from build123d import *

# Parameters (mm, degrees)
EXTRUSION1_DEPTH        = 8
ENL_V_MAT_EXTRU_1_DEPTH = 8


with BuildPart() as part:
    # Esquisse1 → Extrusion1 (new body)
    with BuildSketch(Plane.XY):
        with BuildLine():
            Line((1.5, 0), (16.5, 0))
            ThreePointArc((16.5, 0), (17.560660172, 0.439339828), (18, 1.5))
            Line((18, 1.5), (18, 3.5))
            ThreePointArc((18, 3.5), (17.560660172, 4.560660172), (16.5, 5))
            Line((16.5, 5), (1.5, 5))
            ThreePointArc((1.5, 5), (0.439339828, 4.560660172), (0, 3.5))
            Line((0, 3.5), (0, 1.5))
            ThreePointArc((0, 1.5), (0.439339828, 0.439339828), (1.5, 0))
        make_face()
    extrude(amount=EXTRUSION1_DEPTH)

    # Esquisse2 → Enlèv. mat.-Extru.1 (cut)
    with BuildSketch(Plane.XY.offset(8)):
        with BuildLine():
            Line((2.4, 3.095375723), (15.6, 3.095375723))
            ThreePointArc((15.6, 3.095375723), (15.882842712, 2.978218435), (16, 2.695375723))
            Line((16, 2.695375723), (16, 2.495375723))
            ThreePointArc((16, 2.495375723), (15.882842712, 2.21253301), (15.6, 2.095375723))
            Line((15.6, 2.095375723), (2.4, 2.095375723))
            ThreePointArc((2.4, 2.095375723), (2.117157288, 2.21253301), (2, 2.495375723))
            Line((2, 2.495375723), (2, 2.695375723))
            ThreePointArc((2, 2.695375723), (2.117157288, 2.978218435), (2.4, 3.095375723))
        make_face()
    extrude(amount=-ENL_V_MAT_EXTRU_1_DEPTH, mode=Mode.SUBTRACT)


solid = part.part
Read the model definition and answer for the solid it produces. Units are mm, in the model's axes. A direction names the side the tool comes from. Round coordinates to 2 decimals unless told otherwise and drop trailing zeros. Write each loop counter-clockwise with the first axis right and the second up, starting at its lowest first coordinate (ties: lowest second). Pieces come first, ordered by that corner, then holes.
Q1. The mould has two halves that part along Y. Classify faces 1 (the face through (9, 5, 4)), 2 (the face through (9, 0, 4)), 3 (the face through (9, 3.095, 4)): released by +Y, released by -Y, zero draft, split by the parting line, or undercut.
Values:
face 1: released by +Y
face 2: released by -Y
face 3: undercut
Q2. Find section C-C on y = 2.3. Determine the outline of the cut face in (x, z), and give its area (3 significant figures).
Values:
outline: (0, 0) - (2.05, 0) - (2.05, 8) - (0, 8) - close; (15.95, 0) - (18, 0) - (18, 8) - (15.95, 8) - close
area: 32.8 mm2
Q3. Straight lines are drawn through the part: line 1 (Y direction, x = 10, z = 7.25); line 2 (X direction, y = 3.6, z = 6); line 3 (X direction, y = 0.85, z = 7.25). For each, find the intervals that lie inside material, in ascending order.
Values:
line 1: y = 0 to 2.1, 3.1 to 5
line 2: x = 0 to 18
line 3: x = 0.15 to 17.85
Q4. Find section B-B on z = 1.5. Determine the outline of the cut face in (x, y).
Values:
outline: (0, 1.5) arc R1.5 ccw to (1.5, 0) - (16.5, 0) arc R1.5 ccw to (18, 1.5) - (18, 3.5) arc R1.5 ccw to (16.5, 5) - (1.5, 5) arc R1.5 ccw to (0, 3.5) - close; hole (2, 2.5) arc R0.4 ccw to (2.4, 2.1) - (15.6, 2.1) arc R0.4 ccw to (16, 2.5) - (16, 2.7) arc R0.4 ccw to (15.6, 3.1) - (2.4, 3.1) arc R0.4 ccw to (2, 2.7) - close
Q5. A tool of negligible diameter and unlimited length cuts with its end or side. For faces 4 (the face through (9, 2.095, 4)), 5 (the face through (0, 3, 4)), from which of +Z, -Z, +X, -X, +Y, -Y can it reach the whole face along a straight path? Write none if from no direction.
Values:
face 4: +Z, -Z
face 5: +Z, -Z, -X, +Y, -Y
Q6. A flat-ended cylindrical pin translates along its axis: P1, Ø2, axis at y = 0.5, z = 2, coming from the -X side. Find the tip coordinate at first contact, or state that the pin passes through.
Values:
P1: stops at x = 0
Q7. Find section A-A on x = 8. Determine the outline of the cut face in (y, z), and give its area (3 significant figures).
Values:
outline: (0, 0) - (2.1, 0) - (2.1, 8) - (0, 8) - close; (3.1, 0) - (5, 0) - (5, 8) - (3.1, 8) - close
area: 32.0 mm2
